The drawing under review shows one solid part. Ordinate dimensions are in mm from its lowest x, y, z. Coordinates: 2 decimals unless noted, no trailing zeros. Order: outer loops, then holes, each group sorted by start corner. A loop starts at its lowest first (then second) coordinate and runs counter-clockwise, first axis right, second up.
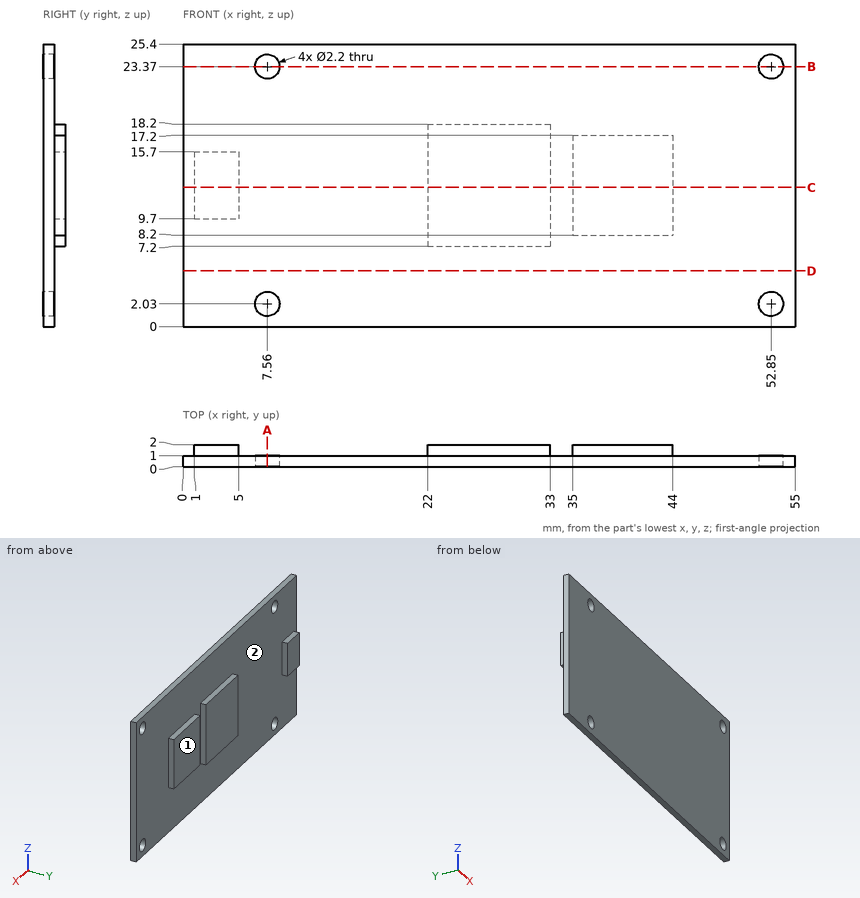
(1) We need section A-A, the plane x = 7.56. Write out the cut boundary in (y, z).
A:
outline: (0, 0) - (1, 0) - (1, 0.93) - (0, 0.93) - close; (0, 3.13) - (1, 3.13) - (1, 22.27) - (0, 22.27) - close; (0, 24.47) - (1, 24.47) - (1, 25.4) - (0, 25.4) - close
(2) We need section D-D, the plane z = 5. Write out the cut boundary in (x, y).
A:
outline: (0, 0) - (55, 0) - (55, 1) - (0, 1) - close
(3) Wall thickness on probe 1 along Z at (x, y) = (7.56, 0.65); probe 2 along X at (y, z) = (0.7, 23.37); probe 3 along X at (y, z) = (1.45, 15.25): over which ranges is each line inside the solid? List them lowest first.
A:
probe 1: z = 0 to 0.93, 3.13 to 22.27, 24.47 to 25.4
probe 2: x = 0 to 6.46, 8.66 to 51.75, 53.95 to 55
probe 3: x = 1 to 5, 22 to 33, 35 to 44
(4) We need section C-C, the plane z = 12.5. Write out the cut boundary in (x, y), and give its area (3 significant figures).
A:
outline: (0, 0) - (55, 0) - (55, 1) - (44, 1) - (44, 2) - (35, 2) - (35, 1) - (33, 1) - (33, 2) - (22, 2) - (22, 1) - (5, 1) - (5, 2) - (1, 2) - (1, 1) - (0, 1) - close
area: 79.0 mm2
(5) Draft analysis for pull direction X (two halves, no side actions). For the marked faces 1 and 2, state which applies: released by +X, released by -X, zero draft, split by the parting line, or undercut.
A:
face 1: zero draft
face 2: undercut
(6) We need section B-B, the plane z = 23.37. Write out the cut boundary in (x, y), and give its area (3 significant figures).
A:
outline: (0, 0) - (6.46, 0) - (6.46, 1) - (0, 1) - close; (8.66, 0) - (51.75, 0) - (51.75, 1) - (8.66, 1) - close; (53.95, 0) - (55, 0) - (55, 1) - (53.95, 1) - close
area: 50.6 mm2
(7) For pin 1 Ø1.5 at (x, z) = (49, 13.5) entering from +Y; pin 2 Ø0.8 at (x, y) = (26, 1.5) entering from -Z; pin 3 Ø0.8 at (x, y) = (3.5, 1.5) entering from +Z, all flat-tipped, find the tip position at first contact; note any pin that passes through.
A:
pin 1: stops at y = 1
pin 2: stops at z = 7.2
pin 3: stops at z = 15.7
